```python
from build123d import *

# Parameters (mm, degrees)
SKETCH_1_W      = 25.6
SKETCH_1_H      = 17
EXTRUDE_1_DEPTH = 44
FILLET_1_R      = 2
SKETCH_2_R      = 3
SKETCH_2_R_2    = 2.1
EXTRUDE_2_DEPTH = 3
FILLET_2_R      = 0.3


with BuildPart() as part:
    # Эскиз1 → Бобышка-Вытянуть1 (new body)
    with BuildSketch(Plane(origin=(0, 0, 0), x_dir=(1, 0, 0), z_dir=(0, 1, 0))):
        Rectangle(SKETCH_1_W, SKETCH_1_H)
    extrude(amount=EXTRUDE_1_DEPTH)

    # Скругление1
    fillet_1_edges = [part.edges().sort_by_distance(p)[0] for p in [
        (12.8, 22, 8.5),
        (-12.8, 22, 8.5),
        (-12.8, 22, -8.5),
        (12.8, 22, -8.5),
    ]]
    fillet(fillet_1_edges, radius=FILLET_1_R)

    # Эскиз2 → Бобышка-Вытянуть2 (add)
    # profile 1 of 2: a face of its own
    with BuildSketch(Plane(origin=(0, 44, 0), x_dir=(1, 0, 0), z_dir=(0, 1, 0))):
        with Locations(Location((6.497670016, 0.020872179, 0), (0, 0, 90))):
            Circle(SKETCH_2_R)
        with Locations(Location((6.497670016, 0.020872179, 0), (0, 0, 270))):
            Circle(SKETCH_2_R_2, mode=Mode.SUBTRACT)
    # profile 2 of 2: a face of its own
    with BuildSketch(Plane(origin=(0, 44, 0), x_dir=(1, 0, 0), z_dir=(0, 1, 0))):
        Polygon((-1.883527831, 0.020872179), (-4.192928907, 4.020872179), (-8.811731061, 4.020872179), (-11.121132138, 0.020872179), (-8.811731061, -3.979127821), (-4.192928907, -3.979127821), align=None)
        Polygon((-3.500108584, 0.020872179), (-5.001219284, 2.620872179), (-8.003440684, 2.620872179), (-9.504551384, 0.020872179), (-8.003440684, -2.579127821), (-5.001219284, -2.579127821), align=None, mode=Mode.SUBTRACT)
    extrude(amount=EXTRUDE_2_DEPTH)

    # Скругление2
    fillet_2_edges = [part.edges().sort_by_distance(p)[0] for p in [
        (6.497670016, 47, 2.979127821),
        (6.497670016, 47, -2.120872179),
        (-3.038228369, 47, 1.979127821),
        (-3.038228369, 47, -2.020872179),
        (-6.502329984, 47, -4.020872179),
        (-9.966431599, 47, -2.020872179),
        (-9.966431599, 47, 1.979127821),
        (-6.502329984, 47, 3.979127821),
        (-4.250663934, 47, 1.279127821),
        (-4.250663934, 47, -1.320872179),
        (-6.502329984, 47, -2.620872179),
        (-8.753996034, 47, -1.320872179),
        (-8.753996034, 47, 1.279127821),
        (-6.502329984, 47, 2.579127821),
    ]]
    fillet(fillet_2_edges, radius=FILLET_2_R)


solid = part.part
```
Geometry check sheet. Reference: the model listing, model coordinates, mm. A direction names the side the tool comes from. Give positions to 0.01 mm unless a question says otherwise; leave off trailing zeros. Loops run counter-clockwise (first coordinate to the right, second up) from the corner with the lowest first, then second, coordinate; pieces in that order, holes last. Notation, with made-up numbers: M 55.5,-0.5 L 104.5,-0.5 A26 cw 104.5,20.5 Z; hole C 46.5,82 d2. An arc over 180 degrees is marked long. Write item = value, one per line. Start each with the question number.
1. Go/stop test with flat-tipped pins: P1, Ø2, axis at x = -7.5, y = 46, coming from the -Z side; P2, Ø4, axis at x = -7, z = 0, coming from the +Y side; P3, Ø0.8, axis at x = -6.5, y = 44.5, coming from the +Z side. Record where each tip stops, or that it passes through.
2. Section check A-A, the plane x = -7. Enter the section's corners in (y, z).
3. Section check B-B, the plane z = -6. Enter the section's corners in (x, y).
4. Thickness scan on probe 1 along X at (y, z) = (45, 0); probe 2 along Y at (x, z) = (7.5, -4); probe 3 along X at (y, z) = (13, -7). Record the ranges inside material, lowest first.
5. Draft check along X on faces 5 (the face through (-3.02, 45.33, -1.99)), 6 (the face through (-7, 45, 3.979)), 7 (the face through (12.8, 22, 0)). Enter one of: +X half, -X half, draft (parallel to the pull), parting line (faces both ways), or undercut.
6. Tool access check on faces 1 (the face through (-3.054, 45.331, 2.007)), 2 (the face through (-3.13, 46.91, -2.01)), 3 (the face through (-4.24, 45.33, -1.3)), 4 (the face through (-9.95, 45.33, -2.05)). Record the directions out of +Z, -Z, +X, -X, +Y, -Y that give a thin tool (end or side, any length) a straight path to the whole face; none if there is none.
7. Section check C-C, the plane x = -1. Enter the section's corners in (y, z), plus the area to 3 significant figures.
Values follow:
q1.P1 = -4.02
q1.P2 = 44
q1.P3 = 3.98
q2.outline = M 0,-8.5 L 44,-8.5 L 44,-4.02 L 46.7,-4.02 A0.3 ccw 47,-3.72 L 47,-2.92 A0.3 ccw 46.7,-2.62 L 44,-2.62 L 44,2.58 L 46.7,2.58 A0.3 ccw 47,2.88 L 47,3.68 A0.3 ccw 46.7,3.98 L 44,3.98 L 44,8.5 L 0,8.5 Z
q3.outline = M -12.8,0 L 12.8,0 L 12.8,44 L -12.8,44 Z
q4.probe_1 = -11.11 to -9.49, -3.51 to -1.9, 3.5 to 4.4, 8.6 to 9.5
q4.probe_2 = 0 to 44
q4.probe_3 = -12.74 to 12.74
q5.face_5 = undercut
q5.face_6 = draft
q5.face_7 = +X half
q6.face_1 = +Z, +Y
q6.face_2 = -Z, +Y
q6.face_3 = +Y
q6.face_4 = -Z, -X, +Y
q7.outline = M 0,-8.5 L 44,-8.5 L 44,8.5 L 0,8.5 Z
q7.area = 748 mm^2
